For this review, take the finished solid that the model builds, in its own axes (mm). Coordinates: 2 decimals unless noted, no trailing zeros. Write each loop counter-clockwise with the first axis right and the second up, starting at its lowest first coordinate (ties: lowest second). Pieces come first, ordered by that corner, then holes.
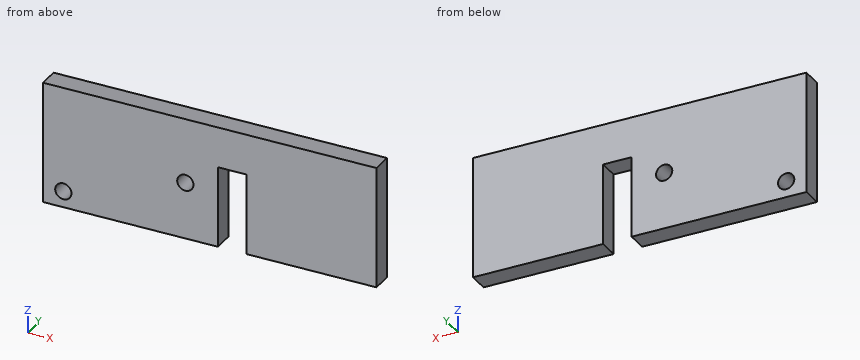
```python
from build123d import *

# Parameters (mm, degrees)
SKETCH1_R           = 2
BOSS_EXTRUDE1_DEPTH = 5


with BuildPart() as part:
    # Sketch1 → Boss-Extrude1 (new body)
    with BuildSketch(Plane(origin=(0, 0, 0), x_dir=(1, 0, 0), z_dir=(0, 1, 0))):
        Polygon((50, 30), (82, 30), (82, 0), (0, 0), (0, 30), (43, 30), (43, 10), (50, 10), align=None)
        with Locations(Location((5, 26, 0), (0, 0, 270))):
            Circle(SKETCH1_R, mode=Mode.SUBTRACT)
        with Locations(Location((35, 16, 0), (0, 0, 270))):
            Circle(SKETCH1_R, mode=Mode.SUBTRACT)
    extrude(amount=-BOSS_EXTRUDE1_DEPTH)


solid = part.part
```
1) Consider section A-A (z = -20.5). Give the boundary of the cut face in (x, y).
2) For L1, parallel to X at y = -1.2, z = -16; L2, parallel to X at y = -3.9, z = -26; L3, parallel to X at y = -3.9, z = -19.25, list the stretches that pass through material, from the lowest coordinate up.
3) Consider section D-D (y = -1.15). Give the boundary of the cut face in (x, z), then the cut area to 3 significant figures.
4) Consider section B-B (x = 35). Give the boundary of the cut face in (y, z), then the cut area to 3 significant figures.
5) Consider section C-C (z = -26). Give the boundary of the cut face in (x, y), then the cut area to 3 significant figures.
6) Clearance check with a flat-ended pin moving along its axis: P1, Ø1.5, axis at x = 45, y = -2.5, coming from the -Z side. State where the tip first meets the part, or that it passes through.
Results:
1. outline: (0, -5) - (43, -5) - (43, 0) - (0, 0) - close; (50, -5) - (82, -5) - (82, 0) - (50, 0) - close
2. L1: x = 0 to 33, 37 to 43, 50 to 82
2. L2: x = 0 to 3, 7 to 43, 50 to 82
2. L3: x = 0 to 43, 50 to 82
3. outline: (0, -30) - (43, -30) - (43, -10) - (50, -10) - (50, -30) - (82, -30) - (82, 0) - (0, 0) - close; hole circle Ø4 at (5, -26); hole circle Ø4 at (35, -16)
3. area: 2,290 mm2
4. outline: (-5, -30) - (0, -30) - (0, -18) - (-5, -18) - close; (-5, -14) - (0, -14) - (0, 0) - (-5, 0) - close
4. area: 130 mm2
5. outline: (0, -5) - (3, -5) - (3, 0) - (0, 0) - close; (7, -5) - (43, -5) - (43, 0) - (7, 0) - close; (50, -5) - (82, -5) - (82, 0) - (50, 0) - close
5. area: 355 mm2
6. P1: stops at z = -10
